```python
from build123d import *

# Parameters (mm, degrees)
BOSS_EXTRUDE1_DEPTH = 25
CUT_EXTRUDE1_REACH  = 31.553
SKETCH3_R           = 1.4


with BuildPart() as part:
    # Sketch1 → Boss-Extrude1 (new body)
    with BuildSketch(Plane.XY):
        with BuildLine():
            Line((-17.6, 0.8), (-9.688838924, 0.8))
            ThreePointArc((-9.688838924, 0.8), (-8.036343261, 1.958278485), (-8.561462594, 3.906765244))
            ThreePointArc((-8.561462594, 3.906765244), (-13.349996928, 14.140943968), (-8.575351799, 24.381609919))
            Line((-8.575351799, 24.381609919), (-11.137608501, 27.438745265))
            ThreePointArc((-11.137608501, 27.438745265), (-11.038357078, 28.565754207), (-9.911348137, 28.466502784))
            Line((-9.911348137, 28.466502784), (-7.349091434, 25.409367438))
            ThreePointArc((-7.349091434, 25.409367438), (-6.981520468, 24.24124721), (-7.54759428, 23.155349554))
            ThreePointArc((-7.54759428, 23.155349554), (0, 2.4), (7.54759428, 23.155349554))
            ThreePointArc((7.54759428, 23.155349554), (6.981520468, 24.24124721), (7.349091434, 25.409367438))
            Line((7.349091434, 25.409367438), (9.911348137, 28.466502784))
            ThreePointArc((9.911348137, 28.466502784), (11.038357078, 28.565754207), (11.137608501, 27.438745265))
            Line((11.137608501, 27.438745265), (8.575351799, 24.381609919))
            ThreePointArc((8.575351799, 24.381609919), (13.349996928, 14.140943968), (8.561462594, 3.906765244))
            ThreePointArc((8.561462594, 3.906765244), (8.036343261, 1.958278485), (9.688838924, 0.8))
            Line((9.688838924, 0.8), (17.6, 0.8))
            Line((17.6, 0.8), (17.6, -0.8))
            Line((17.6, -0.8), (-17.6, -0.8))
            Line((-17.6, -0.8), (-17.6, 0.8))
        make_face()
    extrude(amount=BOSS_EXTRUDE1_DEPTH)

    # Sketch3 → Cut-Extrude1 (cut, up to next)
    with BuildSketch(Plane.XZ.offset(0.8), mode=Mode.PRIVATE) as cut_extrude1_sk1:
        with Locations((-15, 21.8)):
            Circle(SKETCH3_R)
    cut_extrude1_tool1 = extrude(cut_extrude1_sk1.sketch, amount=-CUT_EXTRUDE1_REACH, mode=Mode.PRIVATE) & part.part
    add(cut_extrude1_tool1.solids().sort_by_distance((-15, -0.8, 21.8))[0], mode=Mode.SUBTRACT)
    # Sketch3 → Cut-Extrude1 (cut, up to next)
    with BuildSketch(Plane.XZ.offset(0.8), mode=Mode.PRIVATE) as cut_extrude1_sk2:
        with Locations((15.1, 21.8)):
            Circle(SKETCH3_R)
    cut_extrude1_tool2 = extrude(cut_extrude1_sk2.sketch, amount=-CUT_EXTRUDE1_REACH, mode=Mode.PRIVATE) & part.part
    add(cut_extrude1_tool2.solids().sort_by_distance((15.1, -0.8, 21.8))[0], mode=Mode.SUBTRACT)
    # Sketch3 → Cut-Extrude1 (cut, up to next)
    with BuildSketch(Plane.XZ.offset(0.8), mode=Mode.PRIVATE) as cut_extrude1_sk3:
        with Locations((-15, 2.8)):
            Circle(SKETCH3_R)
    cut_extrude1_tool3 = extrude(cut_extrude1_sk3.sketch, amount=-CUT_EXTRUDE1_REACH, mode=Mode.PRIVATE) & part.part
    add(cut_extrude1_tool3.solids().sort_by_distance((-15, -0.8, 2.8))[0], mode=Mode.SUBTRACT)
    # Sketch3 → Cut-Extrude1 (cut, up to next)
    with BuildSketch(Plane.XZ.offset(0.8), mode=Mode.PRIVATE) as cut_extrude1_sk4:
        with Locations((15.1, 2.8)):
            Circle(SKETCH3_R)
    cut_extrude1_tool4 = extrude(cut_extrude1_sk4.sketch, amount=-CUT_EXTRUDE1_REACH, mode=Mode.PRIVATE) & part.part
    add(cut_extrude1_tool4.solids().sort_by_distance((15.1, -0.8, 2.8))[0], mode=Mode.SUBTRACT)


solid = part.part
```
Verification items for the finished model (mm, model axes). A direction names the side the tool comes from. Give positions to 0.01 mm unless a question says otherwise; leave off trailing zeros. Order: outer loops, then holes, each group sorted by start corner. A loop starts at its lowest first (then second) coordinate and runs counter-clockwise, first axis right, second up. Notation, with made-up numbers: (40, 35) - (97, 35) arc R17 ccw to (97, 45) - close; hole circle Ø2 at (27.25, -5). An arc over 180 degrees is marked (long way). Answer as CSV lines item,"result". Start each with the question number.
Item 1: Section check D-D, the plane z = 10.5. Record the boundary of the cut face in (x, y).
Item 2: Section check C-C, the plane y = 14.15. Record the boundary of the cut face in (x, z), plus the area to 3 significant figures.
Item 3: Access from +Z, -Z, +X, -X, +Y, -Y to the whole of each face (thin tool, end or side, straight path). Record for faces 5 (the face through (0, 2, 25)), 6 (the face through (-9.84, 25.89, 12.32)), 7 (the face through (9.874, 25.932, 12.325)), 8 (the face through (-6.98, 24.26, 12.32)).
Item 4: Material ranges on L1, parallel to Z at x = 15.1, y = -0.4; L2, parallel to X at y = 14.15, z = 16; L3, parallel to Y at x = 0, z = 18.25, recorded low to high.
Item 5: Gauge pin test, flat ends, axial feed: pin 1 (3 mm diameter, centred on x = 15.1, z = 21.8, fed in from +Y); pin 2 (1.7 mm diameter, centred on x = -15, z = 2.8, fed in from +Y); pin 3 (1.5 mm diameter, centred on y = 25.5, z = 17, fed in from -X); pin 4 (5 mm diameter, centred on y = 17.5, z = 20.5, fed in from +X). Record the tip position at first contact, or that the pin passes through.
Item 6: Section check B-B, the plane z = 2.8. Record the boundary of the cut face in (x, y), plus the area to 3 significant figures.
Item 7: Section check A-A, the plane x = 15.1. Record the boundary of the cut face in (y, z).
Item 8: Mould release check, pull along Y, two halves, no side actions. Record for faces 1 (the face through (0, -0.8, 12)), 2 (the face through (14, 0.8, 12)), 3 (the face through (14.07, -0.01, 3.75)), 4 (the face through (8.6, 26.9, 12.3)): released by +Y, released by -Y, zero draft, split by the parting line, or undercut.
Filled in:
1,outline,"(-17.6, -0.8) - (17.6, -0.8) - (17.6, 0.8) - (9.69, 0.8) arc R1.76 cw to (8.56, 3.91) arc R13.35 ccw to (8.58, 24.38) - (11.14, 27.44) arc R0.8 ccw to (9.91, 28.47) - (7.35, 25.41) arc R1.6 ccw to (7.55, 23.16) arc R11.75 cw (long way) to (-7.55, 23.16) arc R1.6 ccw to (-7.35, 25.41) - (-9.91, 28.47) arc R0.8 ccw to (-11.14, 27.44) - (-8.58, 24.38) arc R13.35 ccw to (-8.56, 3.91) arc R1.76 cw to (-9.69, 0.8) - (-17.6, 0.8) - close"
2,outline,"(-13.35, 0) - (-11.75, 0) - (-11.75, 25) - (-13.35, 25) - close; (11.75, 0) - (13.35, 0) - (13.35, 25) - (11.75, 25) - close"
2,area,"80.0 mm^2"
3,face 5,"+Z, +X, -X, +Y, -Y"
3,face 6,"+Z, -Z, -X"
3,face 7,"+Z, -Z, +X"
3,face 8,"+Z, -Z"
4,L1,"0 to 1.4, 4.2 to 20.4, 23.2 to 25"
4,L2,"-13.35 to -11.75, 11.75 to 13.35"
4,L3,"-0.8 to 2.4"
5,pin 1,"y = 0.8"
5,pin 2,"through"
5,pin 3,"x = -10.14"
5,pin 4,"x = 13.32"
6,outline,"(-17.6, -0.8) - (-16.4, -0.8) - (-16.4, 0.8) - (-17.6, 0.8) - close; (-13.6, -0.8) - (13.7, -0.8) - (13.7, 0.8) - (9.69, 0.8) arc R1.76 cw to (8.56, 3.91) arc R13.35 ccw to (8.58, 24.38) - (11.14, 27.44) arc R0.8 ccw to (9.91, 28.47) - (7.35, 25.41) arc R1.6 ccw to (7.55, 23.16) arc R11.75 cw (long way) to (-7.55, 23.16) arc R1.6 ccw to (-7.35, 25.41) - (-9.91, 28.47) arc R0.8 ccw to (-11.14, 27.44) - (-8.58, 24.38) arc R13.35 ccw to (-8.56, 3.91) arc R1.76 cw to (-9.69, 0.8) - (-13.6, 0.8) - close; (16.5, -0.8) - (17.6, -0.8) - (17.6, 0.8) - (16.5, 0.8) - close"
6,area,"179 mm^2"
7,outline,"(-0.8, 0) - (0.8, 0) - (0.8, 1.4) - (-0.8, 1.4) - close; (-0.8, 4.2) - (0.8, 4.2) - (0.8, 20.4) - (-0.8, 20.4) - close; (-0.8, 23.2) - (0.8, 23.2) - (0.8, 25) - (-0.8, 25) - close"
8,face 1,"released by -Y"
8,face 2,"undercut"
8,face 3,"zero draft"
8,face 4,"released by +Y"
